```python
from build123d import *

# Parameters (mm, degrees)
F1_R     = 8
F3_T     = -1.5
F5_D     = 10
F5_DEPTH = 358.0010001
F6_D     = 10


with BuildPart() as f2:
    # F2: sweep along a path in F0
    with BuildLine(Plane.YZ) as f2_path:
        Line((0, 0), (0, 750))
        ThreePointArc((0, 750), (-29.2893218813, 820.7106781187), (-100, 850))
        Line((-100, 850), (-250, 850))
        ThreePointArc((-250, 850), (-320.7106781187, 820.7106781187), (-350, 750))
        Line((-350, 750), (-350, 0))
    # F1 (on Top) → F2 (sweep)
    with BuildSketch(Plane.XY):
        Circle(F1_R)
    sweep(path=f2_path.line)

    # F3
    f3_openings = [f2.faces().sort_by_distance(p)[0] for p in [
        (0, -350, 0),
        (0, 0, 0),
    ]]
    offset(amount=F3_T, openings=f3_openings)

    # F5 (through all, one way)
    with BuildSketch(Plane(origin=(0, 0, 0), x_dir=(1, 0, 0), z_dir=(0, 1, 0))):
        with Locations((0, -425)):
            Circle(F5_D / 2)
    extrude(amount=-F5_DEPTH, mode=Mode.SUBTRACT)

    # F6 (through all)
    with Locations(Plane.XZ):
        with Locations((0, 425)):
            Hole(F6_D / 2)


solid = f2.part
```
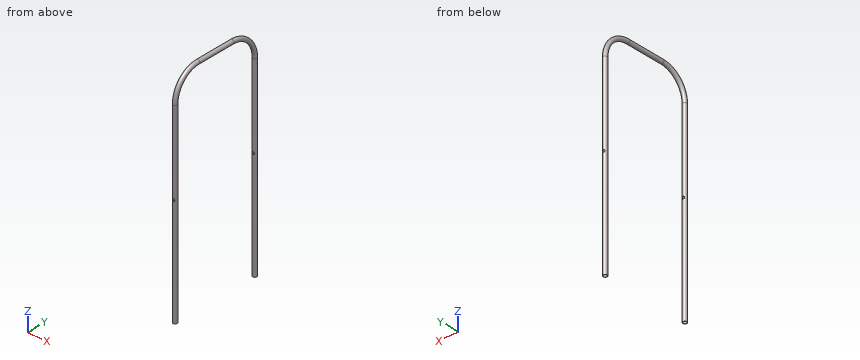
Read the model definition and answer for the solid it produces. Units are mm, in the model's axes. Coordinates: 2 decimals unless noted, no trailing zeros. Write each loop counter-clockwise with the first axis right and the second up, starting at its lowest first coordinate (ties: lowest second). Pieces come first, ordered by that corner, then holes. Notation, with made-up numbers: (25, -8.75) - (62, -8.75) arc R31 cw to (62, 28.25) - close; hole circle Ø4 at (65.25, -7.5). An arc over 180 degrees is marked (long way). Answer as a JSON object with one key per item and string values. Group by question number.
1. A cutting plane is placed at C-C (x = -2). Give the number of separate pieces and of enclosed holes in the cut face, plus the area to 3 significant figures.
2. A cutting plane is placed at B-B (y = -166). Determine the outline of the cut face in (x, z).
3. A cutting plane is placed at A-A (z = 516.5). Determine the outline of the cut face in (x, y), plus the area to 3 significant figures.
4. Consider L1, parallel to Z at x = -0.5, y = -115; L2, parallel to Y at x = 5.5, z = 699; L3, parallel to X at y = -131, z = 850. Determine where each line is inside the solid, lowest interval first. Write a range as [from, to].
5. Each of these flat-tipped pins is pushed along its axis until it touches: P1, Ø6, axis at x = 0, z = 425, coming from the +Y side; P2, Ø2, axis at x = 5, z = 739, coming from the -Y side; P3, Ø1, axis at x = -1, z = 707.5, coming from the +Y side; P4, Ø5, axis at x = 0, y = -240.5, coming from the -Z side. Where does it stop, or does it pass through?
Worked out:
{
 "1": {"separate pieces": "6", "enclosed holes": "0", "area": "6,080 mm²"},
 "2": {"outline": "circle Ø16 at (0, 850); hole circle Ø13 at (0, 850)"},
 "3": {"outline": "circle Ø16 at (0, -350); circle Ø16 at (0, 0); hole circle Ø13 at (0, -350); hole circle Ø13 at (0, 0)", "area": "137 mm²"},
 "4": {"L1": "z = [842.02, 843.52], [856.48, 857.98]", "L2": "y = [-355.81, -353.46], [-346.54, -344.19], [-5.81, -3.46], [3.46, 5.81]", "L3": "x = [-8, -6.5], [6.5, 8]"},
 "5": {"P1": "passes through", "P2": "stops at y = -356.93", "P3": "stops at y = 7.98", "P4": "stops at z = 842"}
}
